from build123d import *

# Parameters (mm, degrees)
SKETCH1_W            = 100
SKETCH1_H            = 80
BOSS_EXTRUDE1_DEPTH  = 5
SKETCH2_W            = 100
SKETCH2_H            = 80
SKETCH2_W_2          = 95
SKETCH2_H_2          = 75
BOSS_EXTRUDE2_DEPTH  = 20
SKETCH3_W            = 25
SKETCH3_H            = 7.5
BOSS_EXTRUDE3_DEPTH  = 20
SKETCH4_W            = 25
SKETCH4_H            = 5
BOSS_EXTRUDE4_DEPTH  = 9
SKETCH5_W            = 8
SKETCH5_H            = 4
BOSS_EXTRUDE5_DEPTH  = 3
FILLET1_R            = 2
FILLET2_R            = 5
FILLET1_OF_MIRROR2_R = 2
CUT_EXTRUDE1_DEPTH   = 132.304988481


with BuildPart() as part:
    # Sketch1 → Boss-Extrude1 (new body)
    with BuildSketch(Plane(origin=(0, 0, 0), x_dir=(1, 0, 0), z_dir=(0, 1, 0))):
        with Locations((50, 40)):
            Rectangle(SKETCH1_W, SKETCH1_H)
    extrude(amount=BOSS_EXTRUDE1_DEPTH)

    # Sketch2 → Boss-Extrude2 (add)
    with BuildSketch(Plane(origin=(0, 5, 0), x_dir=(1, 0, 0), z_dir=(0, 1, 0))):
        with Locations((50, 40)):
            Rectangle(SKETCH2_W, SKETCH2_H)
        with Locations((50, 40)):
            Rectangle(SKETCH2_W_2, SKETCH2_H_2, mode=Mode.SUBTRACT)
    extrude(amount=BOSS_EXTRUDE2_DEPTH)

    # Sketch3 → Boss-Extrude3 (add)
    with BuildSketch(Plane(origin=(0, 5, 0), x_dir=(1, 0, 0), z_dir=(0, 1, 0))):
        with Locations((50, 73.75)):
            Rectangle(SKETCH3_W, SKETCH3_H)
    boss_extrude3 = extrude(amount=BOSS_EXTRUDE3_DEPTH)

    # Sketch4 → Boss-Extrude4 (add)
    with BuildSketch(Plane(origin=(0, 25, 0), x_dir=(1, 0, 0), z_dir=(0, 1, 0))):
        with Locations((50, 72.5)):
            Rectangle(SKETCH4_W, SKETCH4_H)
    boss_extrude4 = extrude(amount=BOSS_EXTRUDE4_DEPTH)

    # Sketch5 → Boss-Extrude5 (add)
    with BuildSketch(Plane(origin=(0, 0, -75), x_dir=(-1, 0, 0), z_dir=(0, 0, -1))):
        with Locations((-50, 32)):
            Rectangle(SKETCH5_W, SKETCH5_H)
    boss_extrude5 = extrude(amount=BOSS_EXTRUDE5_DEPTH)

    # Fillet1
    fillet1_edges = [part.edges().sort_by_distance(p)[0] for p in [
        (50, 30, -78),
        (50, 34, -78),
    ]]
    fillet(fillet1_edges, radius=FILLET1_R - 0.0001)  # a hair under: the kernel refuses the full size

    # Fillet2
    fillet2_edges = [part.edges().sort_by_distance(p)[0] for p in [
        (50, 0, -80),
        (100, 0, -40),
        (50, 0, 0),
        (0, 0, -40),
        (0, 12.5, -80),
        (100, 12.5, -80),
        (100, 12.5, 0),
        (0, 12.5, 0),
    ]]
    fillet(fillet2_edges, radius=FILLET2_R)

    # Mirror2: Boss-Extrude3, Boss-Extrude4, Boss-Extrude5 across plane
    add(boss_extrude3.mirror(Plane.XY.offset(-40)))
    add(boss_extrude4.mirror(Plane.XY.offset(-40)))
    add(boss_extrude5.mirror(Plane.XY.offset(-40)))

    # Fillet1 of Mirror2
    fillet1_of_mirror2_edges = [part.edges().sort_by_distance(p)[0] for p in [
        (50, 30, -2),
        (50, 34, -2),
    ]]
    fillet(fillet1_of_mirror2_edges, radius=FILLET1_OF_MIRROR2_R - 0.0001)  # a hair under: the kernel refuses the full size

    # Sketch6 → Cut-Extrude1 (cut, through all)
    with BuildSketch(Plane(origin=(0, 5, 0), x_dir=(1, 0, 0), z_dir=(0, 1, 0))):
        with BuildLine():
            Line((27.5, 57.120387913), (72.5, 57.120387913))
            ThreePointArc((72.5, 57.120387913), (90, 39.620387913), (72.5, 22.120387913))
            Line((72.5, 22.120387913), (27.5, 22.120387913))
            ThreePointArc((27.5, 22.120387913), (10.000000977, 39.620387913), (27.5, 57.120387913))
        make_face()
    extrude(amount=-CUT_EXTRUDE1_DEPTH, mode=Mode.SUBTRACT)


solid = part.part
Could you check a few things on this model? Use its own coordinates, in mm. A direction names the side the tool comes from. Round coordinates to 2 decimals unless told otherwise and drop trailing zeros. Write each loop counter-clockwise with the first axis right and the second up, starting at its lowest first coordinate (ties: lowest second). Pieces come first, ordered by that corner, then holes. Notation, with made-up numbers: (83.25, 58) - (118.25, 58) arc R29 cw to (118.25, 95) - close; hole circle Ø8 at (64.5, 51). An arc over 180 degrees is marked (long way). Put each result on its own line as item: value. Start each with the question number.
(1) Will these pins go through, and if not, where does the flat tip stop? pin 1 (3.5 mm diameter, centred on y = 32.5, z = -77, fed in from +X); pin 2 (0.5 mm diameter, centred on x = 48.5, z = -75.5, fed in from -Y); pin 3 (4 mm diameter, centred on x = 39.5, y = 2.5, fed in from +Z); pin 4 (8 mm diameter, centred on y = 4, z = -37, fed in from -X).
(2) I need wall thicknesses on probe 1 along X at (y, z) = (8, -9.5); probe 2 along Z at (x, y) = (18.5, 11.5); probe 3 along X at (y, z) = (24, -27.5). Which ranges of each line are inside material? Lowest first, please.
(3) I want a section at D-D, the plane z = -65.5. Please give me the cut outline in (x, y).
(4) I want a section at B-B, the plane x = 34.5. Please give me the cut outline in (y, z), plus the area to 3 significant figures.
(5) Thinking about a two-plate mould opening in X: for faces 6 (the flat face through (50, 3, -22.12)), 7 (the flat face through (50, 34, -72)), 8 (the flat face through (50, 19, -10)), 9 (the flat face through (46, 32, -76)), which applies, released by +X, released by -X, zero draft, split by the parting line, or undercut?
(6) I want a section at C-C, the plane z = -55. Please give me the cut outline in (x, y).
(7) For faces 1 (the flat face through (80, 15, -77.5)), 2 (the cylindrical face through (49.94, 33.43, -77.4)), 3 (the cylindrical face through (89.996, 2.535, -40.005)), 4 (the cylindrical face through (49.94, 30.57, -77.4)), 5 (the flat face through (49, 15, -80)), which set-ups out of +Z, -Z, +X, -X, +Y, -Y let a thin tool reach every point of the face, with its end or its side?
(8) I want a section at A-A, the plane y = 11. Please give me the cut outline in (x, z), plus the area to 3 significant figures.
Here are the results:
1. pin 1: stops at x = 54
1. pin 2: stops at y = 0.01
1. pin 3: stops at z = -0.03
1. pin 4: stops at x = 0
2. probe 1: x = 0 to 2.5, 37.5 to 62.5, 97.5 to 100
2. probe 2: z = -80 to -77.5, -2.5 to 0
2. probe 3: x = 0 to 2.5, 97.5 to 100
3. outline: (0, 5) arc R5 ccw to (5, 0) - (95, 0) arc R5 ccw to (100, 5) - (100, 25) - (97.5, 25) - (97.5, 5) - (2.5, 5) - (2.5, 25) - (0, 25) - close
4. outline: (0, -75) arc R5 ccw to (5, -80) - (25, -80) - (25, -77.5) - (5, -77.5) - (5, -57.12) - (0, -57.12) - close; (0, -22.12) - (5, -22.12) - (5, -2.5) - (25, -2.5) - (25, 0) - (5, 0) arc R5 ccw to (0, -5) - close
4. area: 314 mm^2
5. face 6: undercut
5. face 7: zero draft
5. face 8: undercut
5. face 9: released by -X
6. outline: (0, 5) arc R5 ccw to (5, 0) - (19.15, 0) - (19.15, 5) - (2.5, 5) - (2.5, 25) - (0, 25) - close; (80.85, 0) - (95, 0) arc R5 ccw to (100, 5) - (100, 25) - (97.5, 25) - (97.5, 5) - (80.85, 5) - close
7. face 1: +Y
7. face 2: -Z, +X, -X, +Y
7. face 3: +Y, -Y
7. face 4: -Z, +X, -X
7. face 5: -Z, +X, -X, +Y, -Y
8. outline: (0, -75) arc R5 ccw to (5, -80) - (95, -80) arc R5 ccw to (100, -75) - (100, -5) arc R5 ccw to (95, 0) - (5, 0) arc R5 ccw to (0, -5) - close; hole (2.5, -77.5) - (37.5, -77.5) - (37.5, -70) - (62.5, -70) - (62.5, -77.5) - (97.5, -77.5) - (97.5, -2.5) - (62.5, -2.5) - (62.5, -10) - (37.5, -10) - (37.5, -2.5) - (2.5, -2.5) - close
8. area: 1,230 mm^2
